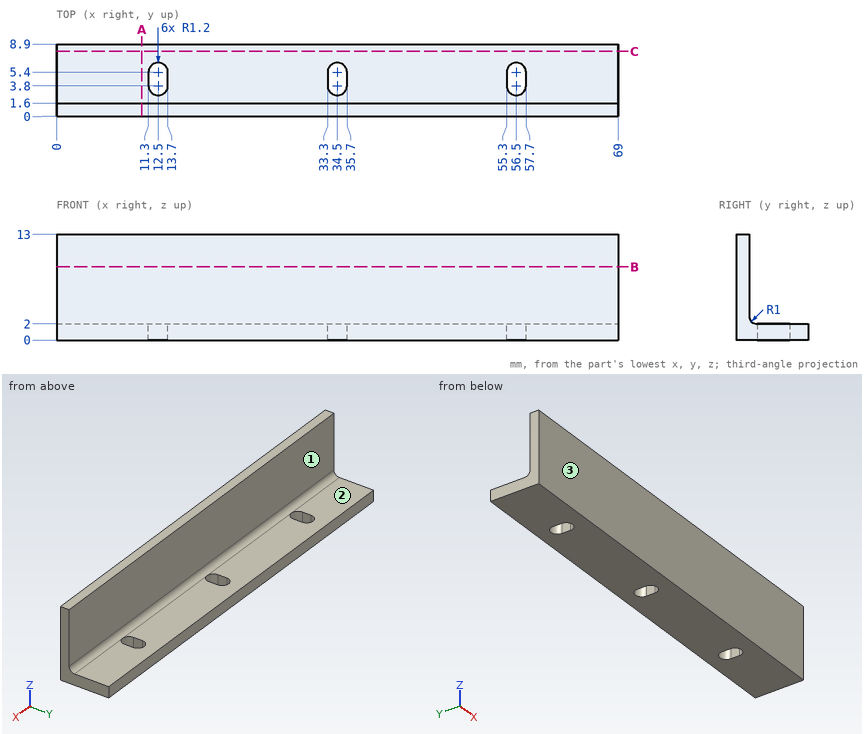
Part print with two shaded views. Sizes in mm from the minimum x, y, z corner. Give positions to 0.01 mm unless a question says otherwise; leave off trailing zeros. Loops run counter-clockwise (first coordinate to the right, second up) from the corner with the lowest first, then second, coordinate; pieces in that order, holes last. Notation, with made-up numbers: (67.25, 89) - (72.25, 89) arc R13 ccw to (72.25, 103) - close; hole circle Ø7 at (1, 31.25). An arc over 180 degrees is marked (long way). Put each result on its own line as item: value.
Q1. Flat gauge pins, fed straight in: pin 1 (5 mm diameter, centred on y = 6.5, z = 5.5, fed in from +X); pin 2 (3 mm diameter, centred on x = 23, y = 5, fed in from +Z). Where does each tip first touch, or does it go through?
Filled in:
pin 1: passes through
pin 2: stops at z = 2
Q2. Slice it at A-A (x = 10.5). Give the cut face in (y, z), plus the area to 3 significant figures.
Filled in:
outline: (0, 0) - (8.9, 0) - (8.9, 2) - (2.6, 2) arc R1 cw to (1.6, 3) - (1.6, 13) - (0, 13) - close
area: 35.6 mm²
Q3. Mould opens along Y. For the marked faces 1, 2 and 3 say: pulls with the +Y half, pulls with the -Y half, needs draft (parallel to the pull), parting line crosses it, or undercut.
Filled in:
face 1: pulls with the +Y half
face 2: needs draft
face 3: pulls with the -Y half
Q4. Probe line 1 along Y through (x, z) = (34, 9); line 2 along Z through (x, y) = (25, 3.75); line 3 along X through (y, z) = (5.75, 0.75). List the from-to ranges inside material, lowest first.
Filled in:
line 1: y = 0 to 1.6
line 2: z = 0 to 2
line 3: x = 0 to 11.35, 13.65 to 33.35, 35.65 to 55.35, 57.65 to 69
Q5. Slice it at C-C (y = 8). Give the cut face in (x, z).
Filled in:
outline: (0, 0) - (69, 0) - (69, 2) - (0, 2) - close
Q6. Slice it at B-B (z = 9). Give the cut face in (x, y), plus the area to 3 significant figures.
Filled in:
outline: (0, 0) - (69, 0) - (69, 1.6) - (0, 1.6) - close
area: 110 mm²
